Can you work these out from the model? Positions are in its coordinate system, mm. Give positions to 0.01 mm unless a question says otherwise; leave off trailing zeros. Loops run counter-clockwise (first coordinate to the right, second up) from the corner with the lowest first, then second, coordinate; pieces in that order, holes last. Notation, with made-up numbers: (-1.5, 41.5) - (47.5, 41.5) arc R4 cw to (47.5, 48.5) - close; hole circle Ø4 at (-34, 62.5). An arc over 180 degrees is marked (long way). Write item = value, one per line.
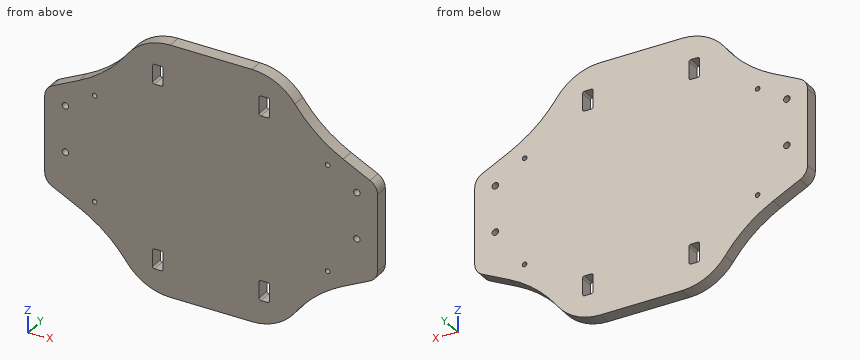
from build123d import *

# Parameters (mm, degrees)
SKETCH2_W           = 8
SKETCH2_H           = 15
SKETCH2_R           = 1.75
SKETCH2_R_2         = 2.425
BOSS_EXTRUDE1_DEPTH = 10
FILLET1_R           = 10
FILLET2_R           = 40
FILLET4_R           = 1.5
FILLET3_R           = 100


with BuildPart() as part:
    # Sketch2 → Boss-Extrude1 (new body)
    with BuildSketch(Plane(origin=(0, 0, 0), x_dir=(1, 0, 0), z_dir=(0, 1, 0))):
        Polygon((70, 95), (-70, 95), (-70, 62.51255638), (-125, 35.036306), (-125, -35.036306), (-70, -62.51255638), (-70, -95), (70, -95), (70, -62.51255638), (125, -35.036306), (125, 35.036306), (70, 62.51255638), align=None)
        with Locations((-40, -69.536306)):
            Rectangle(SKETCH2_W, SKETCH2_H, mode=Mode.SUBTRACT)
        with Locations(Location((-87.5, -40, 0), (0, 0, 270))):
            Circle(SKETCH2_R, mode=Mode.SUBTRACT)
        with Locations(Location((-109.5, -25.761306, 0), (0, 0, 270))):
            Circle(SKETCH2_R_2, mode=Mode.SUBTRACT)
        with Locations((40, -69.536306)):
            Rectangle(SKETCH2_W, SKETCH2_H, mode=Mode.SUBTRACT)
        with Locations(Location((87.5, -40, 0), (0, 0, 270))):
            Circle(SKETCH2_R, mode=Mode.SUBTRACT)
        with Locations(Location((109.5, -25.761306, 0), (0, 0, 270))):
            Circle(SKETCH2_R_2, mode=Mode.SUBTRACT)
        with Locations(Location((-109.5, 9.088694, 0), (0, 0, 270))):
            Circle(SKETCH2_R_2, mode=Mode.SUBTRACT)
        with Locations(Location((-87.5, 40, 0), (0, 0, 270))):
            Circle(SKETCH2_R, mode=Mode.SUBTRACT)
        with Locations((-40, 69.536306)):
            Rectangle(SKETCH2_W, SKETCH2_H, mode=Mode.SUBTRACT)
        with Locations(Location((109.5, 9.088694, 0), (0, 0, 270))):
            Circle(SKETCH2_R_2, mode=Mode.SUBTRACT)
        with Locations((40, 69.536306)):
            Rectangle(SKETCH2_W, SKETCH2_H, mode=Mode.SUBTRACT)
        with Locations(Location((87.5, 40, 0), (0, 0, 270))):
            Circle(SKETCH2_R, mode=Mode.SUBTRACT)
    extrude(amount=BOSS_EXTRUDE1_DEPTH)

    # Fillet1
    fillet1_edges = [part.edges().sort_by_distance(p)[0] for p in [
        (125, 5, 35.036306),
        (-125, 5, 35.036306),
        (-125, 5, -35.036306),
        (125, 5, -35.036306),
    ]]
    fillet(fillet1_edges, radius=FILLET1_R)

    # Fillet2
    # the kernel refuses this fillet: 40 mm, written as the material it takes off along each edge
    with BuildSketch(Plane(origin=(-70, -98.220463011, 95), x_dir=(0, 0, -1), z_dir=(0, 1, 0))) as fillet2_piece_1:
        with BuildLine():
            CenterArc((40, -39.288185204), FILLET2_R, 100.825233866, 79.174766134)
            Line((0, -39.288185204), (-0.8, -39.288185204))
            Line((-0.8, -39.288185204), (-0.8, 0))
            Line((-0.8, 0), (0, 0.8))
            ThreePointArc((0, 0.8), (16.24372181, 0.8), (32.337192493, 0.785763704))
            Line((32.337192493, 0.785763704), (32.48744362, 0))
        make_face()
    extrude(amount=206.440926021, mode=Mode.SUBTRACT)
    with BuildSketch(Plane(origin=(70, -98.220463011, 95), x_dir=(-1, 0, 0), z_dir=(0, 1, 0))) as fillet2_piece_2:
        with BuildLine():
            CenterArc((39.288185204, -40), FILLET2_R, 90, 79.174766134)
            Line((0, -32.48744362), (-0.785763704, -32.337192493))
            ThreePointArc((-0.785763704, -32.337192493), (-0.8, -16.24372181), (-0.8, 0))
            Line((-0.8, 0), (0, 0.8))
            Line((0, 0.8), (39.288185204, 0.8))
            Line((39.288185204, 0.8), (39.288185204, 0))
        make_face()
    extrude(amount=206.440926021, mode=Mode.SUBTRACT)
    with BuildSketch(Plane(origin=(70, -98.220463011, -95), x_dir=(-1, 0, 0), z_dir=(0, 1, 0))) as fillet2_piece_3:
        with BuildLine():
            CenterArc((39.288185204, 40), FILLET2_R, 190.825233866, 79.174766134)
            Line((0, 32.48744362), (-0.785763704, 32.337192493))
            ThreePointArc((-0.785763704, 32.337192493), (-0.8, 16.24372181), (-0.8, 0))
            Line((-0.8, 0), (0, -0.8))
            Line((0, -0.8), (39.288185204, -0.8))
            Line((39.288185204, -0.8), (39.288185204, 0))
        make_face()
    extrude(amount=206.440926021, mode=Mode.SUBTRACT)
    with BuildSketch(Plane(origin=(-70, -98.220463011, -95), x_dir=(0, 0, 1), z_dir=(0, 1, 0))) as fillet2_piece_4:
        with BuildLine():
            CenterArc((40, 39.288185204), FILLET2_R, 180, 79.174766134)
            Line((0, 39.288185204), (-0.8, 39.288185204))
            Line((-0.8, 39.288185204), (-0.8, 0))
            Line((-0.8, 0), (0, -0.8))
            ThreePointArc((0, -0.8), (16.24372181, -0.8), (32.337192493, -0.785763704))
            Line((32.337192493, -0.785763704), (32.48744362, 0))
        make_face()
    extrude(amount=206.440926021, mode=Mode.SUBTRACT)

    # Fillet4
    fillet4_edges = [part.edges().sort_by_distance(p)[0] for p in [
        (36, 5, 62.036306),
        (36, 5, 77.036306),
        (44, 5, 77.036306),
        (44, 5, 62.036306),
        (-36, 5, 62.036306),
        (-44, 5, 62.036306),
        (-44, 5, 77.036306),
        (-36, 5, 77.036306),
        (36, 5, -77.036306),
        (36, 5, -62.036306),
        (44, 5, -62.036306),
        (44, 5, -77.036306),
        (-44, 5, -77.036306),
        (-44, 5, -62.036306),
        (-36, 5, -62.036306),
        (-36, 5, -77.036306),
    ]]
    fillet(fillet4_edges, radius=FILLET4_R)

    # Fillet3
    fillet3_edges = [part.edges().sort_by_distance(p)[0] for p in [
        (70, 5, 62.51255638),
        (-70, 5, 62.51255638),
        (-70, 5, -62.51255638),
        (70, 5, -62.51255638),
    ]]
    fillet(fillet3_edges, radius=FILLET3_R)


solid = part.part
Q1. Imagine slicing it at C-C, the plane x = -56. Write out the boundary of the cut face in (y, z), then the cut area to 3 significant figures.
Output:
outline = (0, -85.99) - (10, -85.99) - (10, 85.99) - (0, 85.99) - close
area = 1,720 mm2
Q2. For pin 1 (5 mm diameter, centred on x = -36.5, y = 5, fed in from +Z); pin 2 (4.5 mm diameter, centred on x = -109.5, z = -9.09, fed in from -Y); pin 3 (4 mm diameter, centred on x = -41, y = 5, fed in from +Z); pin 4 (4 mm diameter, centred on y = 8, z = 40, fed in from +X), each with a flat end and sliding along its axis, tell me the tip position at first contact or that it passes through.
Output:
pin_1 = 94.86
pin_2 = through
pin_3 = 94.13
pin_4 = 119.07
Q3. Imagine slicing it at A-A, the plane y = 7.5. Give the number of separate pieces and of enclosed holes in the cut face, then the cut area to 3 significant figures.
Output:
separate_pieces = 1
enclosed_holes = 12
area = 35,800 mm2
Q4. I need wall thicknesses on L1, parallel to Z at x = -41, y = 3; L2, parallel to Z at x = -38, y = 5.75; L3, parallel to X at y = 7.25, z = 40. Which ranges of each line are inside material? Lowest first, please.
Output:
L1 = -93.65 to -77.04, -62.04 to 62.04, 77.04 to 93.65
L2 = -94.33 to -77.04, -62.04 to 62.04, 77.04 to 94.33
L3 = -115.06 to -89.25, -85.75 to 85.75, 89.25 to 115.06
Q5. Imagine slicing it at B-B, the plane x = -81. Write out the boundary of the cut face in (y, z), then the cut area to 3 significant figures.
Output:
outline = (0, -59.64) - (10, -59.64) - (10, 59.64) - (0, 59.64) - close
area = 1,190 mm2
